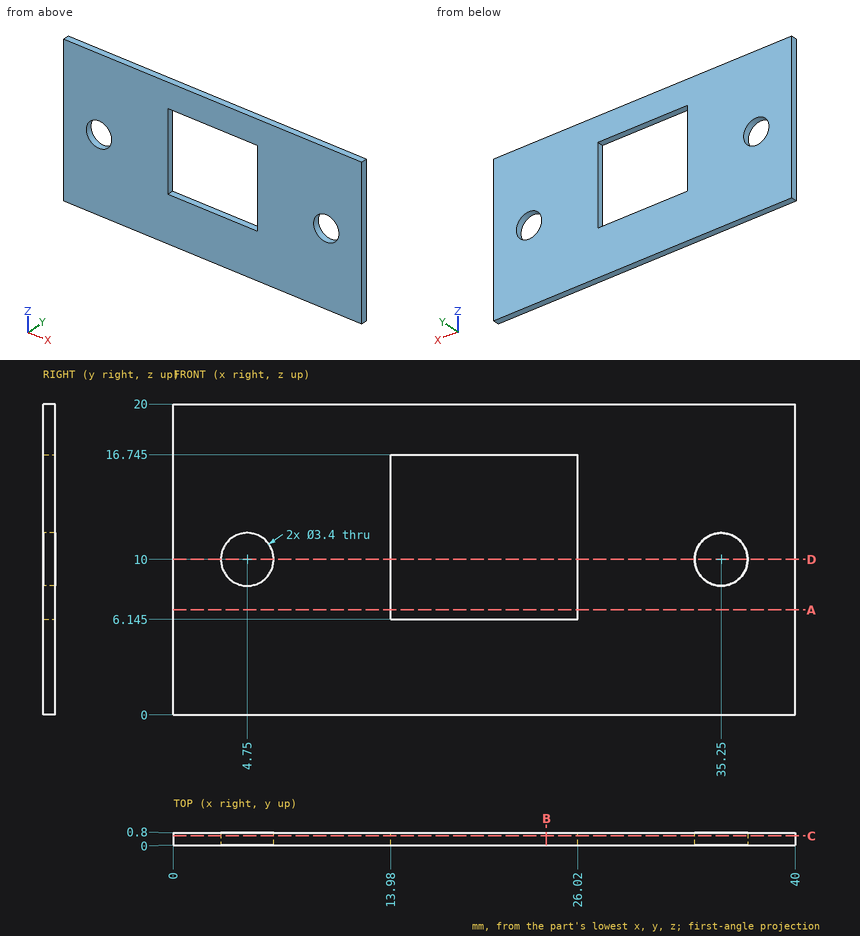
For this review, use the dimensioned drawing (mm, ordinates from the lowest corner) and the shaded views. Round coordinates to 2 decimals unless told otherwise and drop trailing zeros. Order: outer loops, then holes, each group sorted by start corner. A loop starts at its lowest first (then second) coordinate and runs counter-clockwise, first axis right, second up. Notation, with made-up numbers: M -37.5,50.5 L -24.5,50.5 A32 cw -24.5,89.5 Z; hole C -39.75,-19.75 d1. An arc over 180 degrees is marked long. Write each question's results on one line, items separated by ' | '. Start each with the question number.
1. Add section C-C (y = 0.6). State the section outline as (x, z) points (3 decimals).
2. Add section D-D (z = 10). State the section outline as (x, y) points, then the cut area to 3 significant figures.
3. Clearance check with a flat-ended pin moving along its axis: pin 1 Ø2 at (x, z) = (4.75, 10) entering from +Y. State where the tip first meets the part, or that it passes through.
4. To check wall thickness, follow L1, parallel to X at y = 0.1, z = 15; L2, parallel to Z at x = 4.75, y = 0.2; L3, parallel to Z at x = 24, y = 0.15 (3 decimals). State the ranges of each line that lie inside material, in increasing order. Write a range as [from, to].
5. Add section A-A (z = 6.75). State the section outline as (x, y) points, then the cut area to 3 significant figures.
6. Add section B-B (x = 24). State the section outline as (y, z) points (3 decimals), then the cut area to 3 significant figures.
Output values:
1) outline: M 0,0 L 40,0 L 40,20 L 0,20 Z; hole C 4.75,10 d3.4; hole M 13.98,6.145 L 26.02,6.145 L 26.02,16.745 L 13.98,16.745 Z; hole C 35.25,10 d3.4
2) outline: M 0,0 L 3.05,0 L 3.05,0.8 L 0,0.8 Z; M 6.45,0 L 13.98,0 L 13.98,0.8 L 6.45,0.8 Z; M 26.02,0 L 33.55,0 L 33.55,0.8 L 26.02,0.8 Z; M 36.95,0 L 40,0 L 40,0.8 L 36.95,0.8 Z | area: 16.9 mm^2
3) pin 1: through
4) L1: [0, 13.98], [26.02, 40] | L2: [0, 8.3], [11.7, 20] | L3: [0, 6.145], [16.745, 20]
5) outline: M 0,0 L 13.98,0 L 13.98,0.8 L 0,0.8 Z; M 26.02,0 L 40,0 L 40,0.8 L 26.02,0.8 Z | area: 22.4 mm^2
6) outline: M 0,0 L 0.8,0 L 0.8,6.145 L 0,6.145 Z; M 0,16.745 L 0.8,16.745 L 0.8,20 L 0,20 Z | area: 7.52 mm^2
